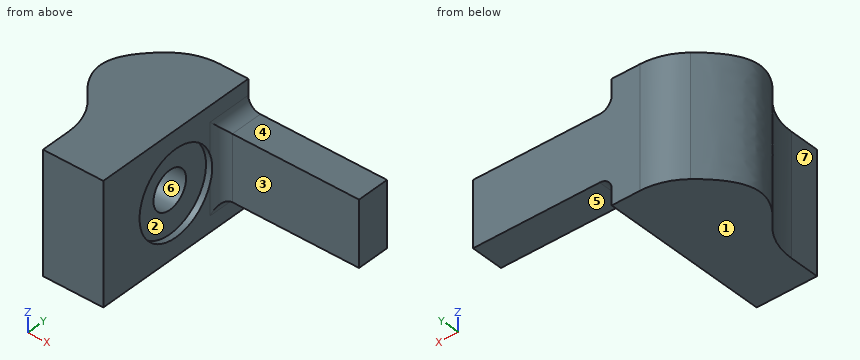
Autodesk Inventor part; units mm, degrees
ref_plane "YZ Plane" through (0, 0, 0) normal (1, 0, 0) x (0, 1, 0)
ref_plane "XZ Plane" through (0, 0, 0) normal (0, 1, 0) x (-1, 0, 0)
ref_plane "XY Plane" through (0, 0, 0) normal (0, 0, 1) x (1, 0, 0)
sketch "Эскиз1" plane through (0, 0, 0) normal (0, 0, 1) x (1, 0, 0)
  spline S0 degree 2 poles (0, -10.75) (-6, -5.75) (0, -0.75) knots -1 -1 -1 0 0 0
  circle A0 centre (31, -8.75) radius 2.1
  circle A1 centre (0.3533, 10.75) radius 2.1
  circle A2 centre (-6.5719, -8.75) radius 2.1
  arc A3 (26, -0.75) -> (0.0249, 0.0543) centre (13, -0.75) ccw
  line L0 (26, -0.75) -> (26, -14.75)
  line L1 (26, -14.75) -> (42.8533, -14.75)
  line L2 (42.8533, -14.75) -> (25.4056, 8.5426)
  arc A4 (25.4056, 8.5426) -> (13, 14.75) centre (13, -0.75) ccw
  line L3 (13, 14.75) -> (-7.8522, 14.75)
  line L4 (-7.8522, 14.75) -> (-8.8, 13.8022)
  arc A5 (-8.8, 13.8022) -> (-9.3554, 12.7353) centre (-7.3858, 12.388) ccw
  line L5 (-9.3554, 12.7353) -> (-9.4563, 12.1627)
  line L6 (-9.4563, 12.1627) -> (-3.6467, 12.1627)
  line L7 (-3.6467, 12.1627) -> (-3.6467, 9.9627)
  line L8 (-3.6467, 9.9627) -> (-9.8443, 9.9627)
  line L9 (-9.8443, 9.9627) -> (-13.8491, -12.75)
  line L10 (-13.8491, -12.75) -> (-7.0093, -12.75)
  line L11 (-7.0093, -12.75) -> (-7.0093, -14.75)
  line L12 (-7.0093, -14.75) -> (0, -14.75)
  line L13 (0, -14.75) -> (0, -11.6512)
  line L14 (1.5, -14.75) -> (26, -14.75)
  line L15 (0.9603, -9.5977) -> (1.5, -10.0794)
  line L16 (1.5, -10.0794) -> (1.5, -14.75)
  line L17 (0.9603, -1.9023) -> (2.3298, -0.75)
  line L18 (2.3298, -0.75) -> (26, -0.75)
  spline S1 degree 3 poles (0.0249, 0.0543) (0.0092, -0.1986) (-0.0544, -0.4464) (-0.2708, -0.9048) (-0.4215, -1.1114) (-0.6069, -1.2843) knots 0 0 0 0 0.5 0.5 1 1 1 1
  spline S2 degree 3 poles (-0.6318, -10.1924) (-0.4418, -10.3706) (-0.2885, -10.5841) (-0.1211, -10.951) (-0.0759, -11.0869) (-0.0153, -11.366) (0, -11.5084) (0, -11.6512) knots 0 0 0 0 0.476947 0.476947 0.738474 0.738474 1 1 1 1
  spline S3 degree 2 poles (-0.6318, -10.1924) (-5.3806, -5.7383) (-0.6069, -1.2843) knots -0.944242 -0.944242 -0.944242 -0.053426 -0.053426 -0.053426
  line L19 (1.5, -14.75) -> (6.5, -14.75)
  line L20 (6.5, -14.75) -> (6.5, -0.75)
  spline S4 degree 5 poles (0.9603, -9.5977) (0.5187, -9.2297) (0.0945, -8.8388) (-0.3025, -8.4229) (-0.9009, -7.6836) (-1.3123, -6.8331) (-1.4364, -6.4831) (-1.5637, -5.75) (-1.4364, -5.0169) (-1.3123, -4.6669) (-0.9009, -3.8164) (-0.3025, -3.0771) (0.0945, -2.6612) (0.5187, -2.2703) (0.9603, -1.9023) knots 0 0 0 0 0 0 0.305403 0.305403 0.305403 0.5 0.5 0.5 0.694597 0.694597 0.694597 1 1 1 1 1 1
  point P0 (0, 0)
  dimension "d0" = 1.5
  dimension "d2" = 1.5
  dimension "d12" = 5
extrude "Выдавливание1" add sketch "Эскиз1" against normal blind 10 contours L20 L14 L16 L15 S4 L17 L18
fillet "Сопряжение2" radius 5 2 edges at (1.5, -10.0794, -5) (2.3298, -0.75, -5)
fillet_without_effect "Сопряжение3"
sketch "Эскиз3" plane through (6.5, -14.75, 0) normal (1, 0, 0) x (0, 0, -1)
  line L0 (0, 0) -> (0, 14)
  line L1 (0, 0) -> (10, 0)
  line L2 (10, 14) -> (10, 0)
  line L3 (0, 14) -> (10, 14)
  line L4 (0, 14) -> (10, 14)
  line L5 (5, 14) -> (5, 0)
  line L6 (0, 0) -> (10, 0)
  circle A0 centre (5, 7) radius 1.575
  point P0 (0, 14.75)
  dimension "d13" = 3.15
extrude "Выдавливание3" cut sketch "Эскиз3" against normal blind 5 contours A0 L5 | L5 A0
chamfer "Фаска1" distance 0.7 angle 45 1 edges at (1.5, -7.75, -3.425)
sketch "Эскиз4" plane through (6.5, -14.75, 0) normal (1, 0, 0) x (0, 0, -1)
  line L0 (9, 14) -> (10, 14)
  line L1 (10, 0) -> (10, 14)
  line L2 (0, 0) -> (10, 0)
  line L3 (0, 14) -> (0, 0)
  line L4 (0, 14) -> (1, 14)
  circle A0 centre (5, 7) radius 2.1
  line L5 (7.7, 11.3) -> (2.3, 11.3)
  line L6 (2.3, 11.3) -> (2.3, 14.3)
  line L7 (2.3, 14.3) -> (-0.3, 14.3)
  line L8 (-0.3, 14.3) -> (-0.3, -0.3)
  line L9 (-0.3, -0.3) -> (10.3, -0.3)
  line L10 (10.3, -0.3) -> (10.3, 14.3)
  line L11 (10.3, 14.3) -> (7.7, 14.3)
  line L12 (7.7, 14.3) -> (7.7, 11.3)
  line L13 (0, 14) -> (10, 14)
  line L14 (1, 10) -> (1, 14)
  line L15 (9, 10) -> (1, 10)
  line L16 (9, 14) -> (9, 10)
  point P0 (0, 14.75)
  point P1 (2, 14)
  point P2 (8, 14)
  point P3 (7.7, 14)
  point P4 (2.3, 14)
extrude "Выдавливание4" add sketch "Эскиз4" along normal blind 11.5 contours L12 L5 L6 L13
fillet "Сопряжение4" radius 1 3 edges at (6.5, -2.1, -7.7) (6.5, -3.45, -5) (6.5, -2.1, -2.3)
sketch "Эскиз5" plane through (6.5, -14.75, 0) normal (1, 0, 0) x (0, 0, -1)
  circle A0 centre (5, 7) radius 1.575
  line L0 (8.7, 10.3) -> (8.7, 14)
  line L1 (1.3, 10.3) -> (8.7, 10.3)
  line L2 (1.3, 14) -> (1.3, 10.3)
  line L3 (0, 14) -> (1.3, 14)
  line L4 (0, 0) -> (0, 14)
  line L5 (0, 0) -> (10, 0)
  line L6 (10, 14) -> (10, 0)
  line L7 (8.7, 14) -> (10, 14)
  circle A1 centre (5, 7) radius 1.575
  circle A2 centre (5, 7) radius 3.5
  point P0 (0, 14.75)
  point P1 (3.8338, 10.3)
  point P2 (6.1662, 10.3)
  dimension "d23" = 7
extrude "Выдавливание5" cut sketch "Эскиз5" along normal mid plane 1 contours A0 | A2 L1 | L1 A2
properties part number "upor"
CAD build for the part. Positions are in the model's coordinates, mm. Face numbers are marked on the shaded views. A direction names the side the tool comes from. Coordinates: 2 decimals unless noted, no trailing zeros. Write each loop counter-clockwise with the first axis right and the second up, starting at its lowest first coordinate (ties: lowest second). Pieces come first, ordered by that corner, then holes. Notation, with made-up numbers: M 53.5,11 L 96.5,11 A20 cw 96.5,23 Z; hole C 49,-29 d6. An arc over 180 degrees is marked long. Return JSON: item names as keys, results as strings.
Item 1: Two-plate mould, pull along Z, no slides. Class the marked faces 1, 2 and 3: +Z half, -Z half, draft (parallel to the pull), parting line (faces both ways), or undercut.
Findings below:
{"face 1": "-Z half", "face 2": "undercut", "face 3": "draft"}
Item 2: Which spindle directions (+Z, -Z, +X, -X, +Y, -Y) get a long thin tool onto all of the face, cutting with end or side? Do the marked faces 4, 5, 6 and 7. Say none if no direction does.
Findings below:
{"face 4": "+Z, +X, +Y, -Y", "face 5": "-Z, +X, +Y, -Y", "face 6": "+X", "face 7": "+Z, -Z, -X, -Y"}
Item 3: Drop flat-ended pins along their axis: pin 1 Ø1.4 at (y, z) = (-8, -4.5) entering from +X; pin 2 Ø2.5 at (x, z) = (12, -5.5) entering from -Y; pin 3 Ø1.5 at (x, y) = (10.5, -5.5) entering from +Z; pin 4 Ø1.2 at (y, z) = (-13.5, -3.5) entering from -X. Give the stop position or say it passes through.
Findings below:
{"pin 1": "stops at x = 1.88", "pin 2": "stops at y = -3.45", "pin 3": "passes through", "pin 4": "stops at x = 1.5"}
Item 4: Slice it at A-A, the plane x = 9.75. Write the cut outline in (y, z).
Findings below:
{"outline": "M -3.45,-7.7 L -0.75,-7.7 L -0.75,-2.3 L -3.45,-2.3 Z"}
Item 5: Probe line 1 (Y direction, x = 6.4, z = -5); line 2 (Z direction, x = 6.45, y = -7.75); line 3 (Y direction, x = 14.75, z = -3). List the from-to ranges inside material, lowest first. Write a range as from..to.
Findings below:
{"line 1": "y = -14.75..-11.25, -4.25..-0.75", "line 2": "z = -10..-8.5, -1.5..0", "line 3": "y = -3.45..-0.75"}
